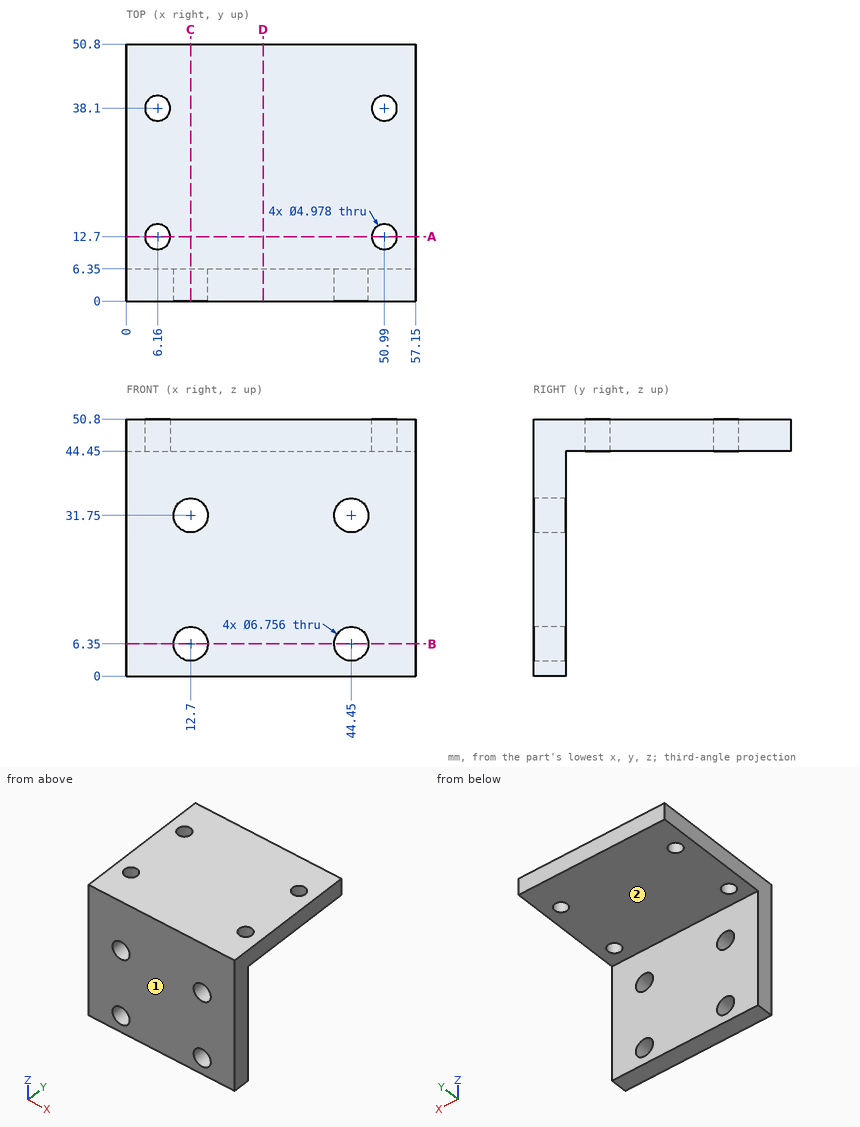
For this review, use the dimensioned drawing (mm, ordinates from the lowest corner) and the shaded views. A direction names the side the tool comes from. Round coordinates to 2 decimals unless told otherwise and drop trailing zeros. Write each loop counter-clockwise with the first axis right and the second up, starting at its lowest first coordinate (ties: lowest second). Pieces come first, ordered by that corner, then holes. Notation, with made-up numbers: M -21.75,50.25 L 33.25,50.25 A7 cw 33.25,58.25 Z; hole C -33.5,52.25 d9. An arc over 180 degrees is marked long. Write item = value, one per line. Start each with the question number.
(1) For line 1 along X through (y, z) = (2, 31.75); line 2 along X through (y, z) = (12, 46); line 3 along Z through (x, y) = (12, 5.5) (1 decimal), list the stretches that pass through material, from the lowest coordinate up.
(2) We need section B-B (z = 6.35). Give the boundary of the cut face in (x, y).
(3) We need section A-A (y = 12.7). Give the boundary of the cut face in (x, z).
(4) We need section D-D (x = 27). Give the boundary of the cut face in (y, z).
(5) Clearance check with flat-ended pins moving along their axes: pin 1 Ø9 at (x, z) = (44.45, 6.35) entering from +Y; pin 2 Ø8 at (x, y) = (50.99, 12.7) entering from -Z. State where each tip first meets the part, or that it passes through.
(6) We need section C-C (x = 12.7). Give the boundary of the cut face in (y, z), then the cut area to 3 significant figures.
(7) For the marked faces 1 and 2, list the 3-axis set-ups (+Z, -Z, +X, -X, +Y, -Y) from which the entire face can be reached by the end or side of a thin tool; tool diameter is ignored.
Results found:
q1.line_1 = 0 to 9.32, 16.08 to 41.07, 47.83 to 57.15
q1.line_2 = 0 to 3.77, 8.55 to 48.6, 53.38 to 57.15
q1.line_3 = 0 to 3, 9.7 to 28.4, 35.1 to 50.8
q2.outline = M 0,0 L 9.32,0 L 9.32,6.35 L 0,6.35 Z; M 16.08,0 L 41.07,0 L 41.07,6.35 L 16.08,6.35 Z; M 47.83,0 L 57.15,0 L 57.15,6.35 L 47.83,6.35 Z
q3.outline = M 0,44.45 L 3.67,44.45 L 3.67,50.8 L 0,50.8 Z; M 8.65,44.45 L 48.5,44.45 L 48.5,50.8 L 8.65,50.8 Z; M 53.48,44.45 L 57.15,44.45 L 57.15,50.8 L 53.48,50.8 Z
q4.outline = M 0,0 L 6.35,0 L 6.35,44.45 L 50.8,44.45 L 50.8,50.8 L 0,50.8 Z
q5.pin_1 = 6.35
q5.pin_2 = 44.45
q6.outline = M 0,0 L 6.35,0 L 6.35,2.97 L 0,2.97 Z; M 0,9.73 L 6.35,9.73 L 6.35,28.37 L 0,28.37 Z; M 0,35.13 L 6.35,35.13 L 6.35,44.45 L 50.8,44.45 L 50.8,50.8 L 0,50.8 Z
q6.area = 519 mm²
q7.face_1 = +Z, -Z, +X, -X, -Y
q7.face_2 = -Z, +X, -X, +Y
